The model under review builds one solid part; all positions refer to its coordinate system, in mm. A direction names the side the tool comes from. Coordinates: 2 decimals unless noted, no trailing zeros. Loops run counter-clockwise (first coordinate to the right, second up) from the corner with the lowest first, then second, coordinate; pieces in that order, holes last. Notation, with made-up numbers: M 29.25,30.25 L 73.25,30.25 A23 ccw 73.25,56.25 Z; hole C -22.5,57 d5. An arc over 180 degrees is marked long. Write item = value, one per line. Start each with the question number.
Q1. For faces 1 (the face through (0, 21, 36)), 2 (the face through (13.5, -2, -1)), 3 (the face through (-7.5, 67, -10.8)), 4 (the face through (9, 33, -24)), 5 (the face through (9, 66, -26)), list the 3-axis set-ups (+Z, -Z, +X, -X, +Y, -Y) from which the entire face can be reached by the end or side of a thin tool; tool diameter is ignored.
Q2. Mouldability with a two-part tool opening along X and no side actions: class faces 6 (the face through (0, 42, 38)), 7 (the face through (0, 34, -39)), 8 (the face through (-0.297, -1.521, -61.497)), 9 (the face through (7.599, -1.521, 46.194)) as released by +X, released by -X, zero draft, split by the parting line, or undercut.
Q3. We need section D-D on z = -2.5. Give the boundary of the cut face in (x, y), and give its area (3 significant figures).
Q4. We need section C-C on y = 45.5. Give the boundary of the cut face in (x, z).
Q5. We need section A-A on z = -56. Give the boundary of the cut face in (x, y).
Q6. Clearance check with flat-ended pins moving along their axes: pin 1 Ø1 at (x, y) = (6, 28.5) entering from -Z; pin 2 Ø4.5 at (x, z) = (0, 56) entering from -Y; pin 3 Ø8 at (y, z) = (49, 24.5) entering from -X; pin 4 Ø6 at (x, y) = (-1.5, 26) entering from +Z. State where each tip first meets the part, or that it passes through.
Q7. We need section B-B on x = 0. Give the boundary of the cut face in (y, z), and give its area (3 significant figures).
Q8. Wall thickness on probe 1 along Z at (x, y) = (0, 7.5); probe 2 along Z at (x, y) = (9.75, 12.5); probe 3 along Z at (x, y) = (-8, -1.55): over which ranges is each line inside the solid? List them lowest first.
Autodesk Inventor part; units mm, degrees
ref_plane "YZ Plane" through (0, 0, 0) normal (1, 0, 0) x (0, 1, 0)
ref_plane "XZ Plane" through (0, 0, 0) normal (0, 1, 0) x (-1, 0, 0)
ref_plane "XY Plane" through (0, 0, 0) normal (0, 0, 1) x (1, 0, 0)
sketch "Sketch1" plane through (0, 0, 0) normal (0, 1, 0) x (-1, 0, 0)
  line L0 (-7, -36) -> (7, -36)
  line L1 (7, -36) -> (7, 36)
  line L2 (7, 36) -> (-7, 36)
  line L3 (-7, 36) -> (-7, -36)
  line L4 (-7, -36) -> (7, 36) construction
  line L5 (7, -36) -> (-7, 36) construction
  line L6 (-10, -39) -> (10, -39)
  line L7 (10, -39) -> (10, 39)
  line L8 (10, 39) -> (-10, 39)
  line L9 (-10, 39) -> (-10, -39)
  line L10 (-10, -39) -> (10, 39) construction
  line L11 (10, -39) -> (-10, 39) construction
  point P0 (0, 0)
  dimension "d0" = 14
  dimension "d1" = 72
  dimension "d2" = 20
  dimension "d3" = 78
extrude "Extrusion1" add sketch "Sketch1" along normal blind 42
sketch "Sketch2" plane through (10, 0, 39) normal (1, 0, 0) x (0, 0, -1)
  line L0 (78, 42) -> (0, 42)
  line L1 (12, 5) -> (63, 5)
  line L2 (12, 5) -> (12, 42)
  line L3 (63, 5) -> (63, 42)
  point P0 (39, 0)
  point P1 (39, 42)
  dimension "d6" = 78
  dimension "d7" = 51
extrude "Extrusion2" cut sketch "Sketch2" against normal blind 10
sketch "Sketch3" plane through (0, 42, 0) normal (0, 1, 0) x (1, 0, 0)
  line L0 (-10, 39) -> (-10, -39)
  line L1 (10, 39) -> (-10, 39)
  line L2 (10, 24) -> (10, 39)
  line L3 (-7, 36) -> (7, 36)
  line L4 (7, 36) -> (7, 24)
  line L5 (7, 24) -> (10, 24)
  line L6 (10, -39) -> (10, -27)
  line L7 (10, -27) -> (7, -27)
  line L8 (-7, 36) -> (-7, -36)
  line L9 (-7, -39) -> (-7, 36)
  line L10 (-10, -39) -> (-7, -39)
  line L11 (7, -39) -> (7, -27)
  line L12 (10, -39) -> (7, -39)
  point P0 (0, 0)
extrude "Extrusion3" add sketch "Sketch3" along normal blind 25
sketch "Sketch4" plane through (0, 0, 0) normal (0, -1, 0) x (1, 0, 0)
  line L0 (10, 39) -> (10, -39)
  line L1 (-10, 39) -> (10, 39)
  line L2 (-10, -39) -> (-10, 39)
  line L3 (10, -39) -> (-10, -39)
  point P0 (0, 0)
extrude "Extrusion4" add sketch "Sketch4" along normal blind 3
sketch "Sketch5" plane through (0, -3, 0) normal (0, -1, 0) x (1, 0, 0)
  circle A0 centre (-8, -48) radius 1.85
  circle A1 centre (0, -56) radius 1.85
  circle A2 centre (8, -48) radius 1.85 construction
  circle A3 centre (-8, 48) radius 1.85
  circle A4 centre (0, 56) radius 1.85
  circle A5 centre (8, 48) radius 1.85
  arc A6 (-13.5, -48) -> (13.5, -48) centre (0, -48) ccw
  circle A7 centre (8, -48) radius 1.85
  arc A8 (13.5, 48) -> (-13.5, 48) centre (0, 48) ccw
  line L0 (13.5, -48) -> (13.5, 48)
  line L1 (-13.5, 48) -> (-13.5, -48)
  point P0 (0, 0)
extrude "Extrusion5" add sketch "Sketch5" against normal blind 3
sketch "Sketch6" plane through (0, 67, 0) normal (0, 1, 0) x (1, 0, 0)
  line L0 (10, -39) -> (10, -27)
  line L1 (10, -27) -> (7, -27)
  line L2 (7, -27) -> (7, -39)
  line L3 (7, -39) -> (10, -39)
  point P0 (0, 0)
extrude "Extrusion6" cut sketch "Sketch6" against normal blind 20
fillet "Fillet1" radius 5 4 edges at (8.5, 47, 27) (8.5, 67, -24) (-8.5, 67, 39) (8.5, 47, 39)
properties part number "Phone Mount 2"
Returned:
q1.face_1 = +Y
q1.face_2 = +Z, -Z, +X, +Y, -Y
q1.face_3 = +Z, -Z, +X, -X, +Y
q1.face_4 = +X, +Y
q1.face_5 = +Z, +X, +Y
q2.face_6 = undercut
q2.face_7 = zero draft
q2.face_8 = split by the parting line
q2.face_9 = undercut
q3.outline = M -13.5,-3 L 13.5,-3 L 13.5,0 L 10,0 L 10,5 L 7,5 L 7,0 L -7,0 L -7,67 L -10,67 L -10,0 L -13.5,0 Z
q3.area = 297 mm^2
q4.outline = M -10,-39 L 10,-39 L 10,-24 L 7,-24 L 7,-36 L -7,-36 L -7,39 L -10,39 Z; M 7,28.43 L 10,28.43 L 10,37.57 L 7,37.57 Z
q5.outline = M -10.87,-3 L -1.85,-3 L -1.85,0 L -10.87,0 Z; M 1.85,-3 L 10.87,-3 L 10.87,0 L 1.85,0 Z
q6.pin_1 = -39
q6.pin_2 = -3
q6.pin_3 = -10
q6.pin_4 = 39
q7.outline = M -3,-61.5 L 0,-61.5 L 0,-57.85 L -3,-57.85 Z; M -3,-54.15 L 0,-54.15 L 0,-39 L 67,-39 L 67,-36 L 0,-36 L 0,36 L 42,36 L 42,39 L 0,39 L 0,54.15 L -3,54.15 Z; M -3,57.85 L 0,57.85 L 0,61.5 L -3,61.5 Z
q7.area = 674 mm^2
q8.probe_1 = -39 to -36, 36 to 39
q8.probe_2 = -39 to -24, 27 to 39
q8.probe_3 = -58.87 to -49.85, -46.15 to 46.15, 49.85 to 58.87
